Verification items for the finished model (mm, model axes). Coordinates: 2 decimals unless noted, no trailing zeros. Order: outer loops, then holes, each group sorted by start corner. A loop starts at its lowest first (then second) coordinate and runs counter-clockwise, first axis right, second up. Notation, with made-up numbers: (49, -27) - (75, -27) arc R25 cw to (75, 7) - close; hole circle Ø10 at (10.5, 73). An arc over 180 degrees is marked (long way). Answer as CSV lines item,"result". Start each with the question number.
1. Material ranges on L1, parallel to Z at x = 38.1, y = 10.25; L2, parallel to Y at x = -38, z = -1; L3, parallel to X at y = 13, z = 12, recorded low to high. Write a range as [from, to].
2. Go/stop test with flat-tipped pins: pin 1 (4 mm diameter, centred on x = 7.5, z = 10, fed in from -Y); pin 2 (11.5 mm diameter, centred on x = -38.1, y = 12.7, fed in from -Z). Record where each tip stops, or that it passes through.
3. Section check C-C (y = 7.5). Record the cut outline in (x, z), and give its area (3 significant figures).
4. Section check B-B (z = 0). Record the cut outline in (x, y), and give its area (3 significant figures).
5. Mould release check, pull along Y, two halves, no side actions. Record for faces 1 (the cylindrical face through (-31.756, 12.979, -0.267)), 2 (the flat face through (1, 25.4, 0)), 3 (the flat face through (-50.8, 13, 0)): pulls with the +Y half, pulls with the -Y half, needs draft (parallel to the pull), parting line crosses it, or undercut.
6. Section check D-D (z = -15). Record the cut outline in (x, y).
7. Section check A-A (x = 38.1). Record the cut outline in (y, z), and give its area (3 significant figures).
Autodesk Inventor part; units mm, degrees
ref_plane "YZ Plane" through (0, 0, 0) normal (1, 0, 0) x (0, 1, 0)
ref_plane "XZ Plane" through (0, 0, 0) normal (0, 1, 0) x (-1, 0, 0)
ref_plane "XY Plane" through (0, 0, 0) normal (0, 0, 1) x (1, 0, 0)
sketch "Sketch1" plane through (0, 0, 0) normal (0, 1, 0) x (-1, 0, 0)
  line L0 (-50.8, -19.05) -> (50.8, -19.05)
  line L1 (50.8, -19.05) -> (50.8, 19.05)
  line L2 (50.8, 19.05) -> (-50.8, 19.05)
  line L3 (-50.8, 19.05) -> (-50.8, -19.05)
  line L4 (-50.8, -19.05) -> (50.8, 19.05) construction
  line L5 (50.8, -19.05) -> (-50.8, 19.05) construction
  point P0 (0, 0)
  dimension "d0" = 38.1
  dimension "d1" = 101.6
extrude "Extrusion1" add sketch "Sketch1" along normal blind 25.4
sketch "Sketch2" plane through (50.8, 0, -19.05) normal (0, 0, -1) x (-1, 0, 0)
  line L0 (101.6, 0) -> (101.6, 25.4)
  line L1 (101.6, 12.7) -> (0, 12.7) construction
  line L2 (0, 0) -> (0, 25.4)
  circle A0 centre (88.9, 12.7) radius 6.35
  point P0 (50.8, 0)
  dimension "d4" = 12.7
  dimension "d5" = 12.7
extrude "Extrusion2" cut sketch "Sketch2" against normal through all
sketch "Sketch3" plane through (0, 0, 0) normal (0, -1, 0) x (1, 0, 0)
  line L0 (50.8, 19.05) -> (50.8, -19.05)
  line L1 (50.8, 0) -> (-50.8, 0) construction
  line L2 (-50.8, -19.05) -> (-50.8, 19.05)
  circle A0 centre (38.1, 0) radius 6.35
  point P0 (0, 0)
  dimension "d8" = 12.7
  dimension "d9" = 12.7
extrude "Extrusion3" cut sketch "Sketch3" against normal blind 25.4
properties part number "tie rod"
Evaluation:
1,L1,"z = [-19.05, -6.35], [6.35, 19.05]"
1,L2,"y = [0, 6.35], [19.05, 25.4]"
1,L3,"x = [-50.8, -44.44], [-31.76, 50.8]"
2,pin 1,"stops at y = 0"
2,pin 2,"passes through"
3,outline,"(-50.8, -19.05) - (-41.74, -19.05) - (-41.74, 19.05) - (-50.8, 19.05) - close; (-34.46, -19.05) - (50.8, -19.05) - (50.8, 19.05) - (-34.46, 19.05) - close; hole circle Ø12.7 at (38.1, 0)"
3,area,"3,470 mm²"
4,outline,"(-50.8, 0) - (31.75, 0) - (31.75, 25.4) - (-50.8, 25.4) - close; (44.45, 0) - (50.8, 0) - (50.8, 25.4) - (44.45, 25.4) - close; hole circle Ø12.7 at (-38.1, 12.7)"
4,area,"2,130 mm²"
5,face 1,"undercut"
5,face 2,"pulls with the +Y half"
5,face 3,"needs draft"
6,outline,"(-50.8, 0) - (50.8, 0) - (50.8, 25.4) - (-50.8, 25.4) - close; hole circle Ø12.7 at (-38.1, 12.7)"
7,outline,"(0, -19.05) - (25.4, -19.05) - (25.4, -6.35) - (0, -6.35) - close; (0, 6.35) - (25.4, 6.35) - (25.4, 19.05) - (0, 19.05) - close"
7,area,"645 mm²"
